Here's the drawing with two shaded views (mm, measured from the low corner). I have some questions. Round coordinates to 2 decimals unless told otherwise and drop trailing zeros. Write each loop counter-clockwise with the first axis right and the second up, starting at its lowest first coordinate (ties: lowest second). Pieces come first, ordered by that corner, then holes.
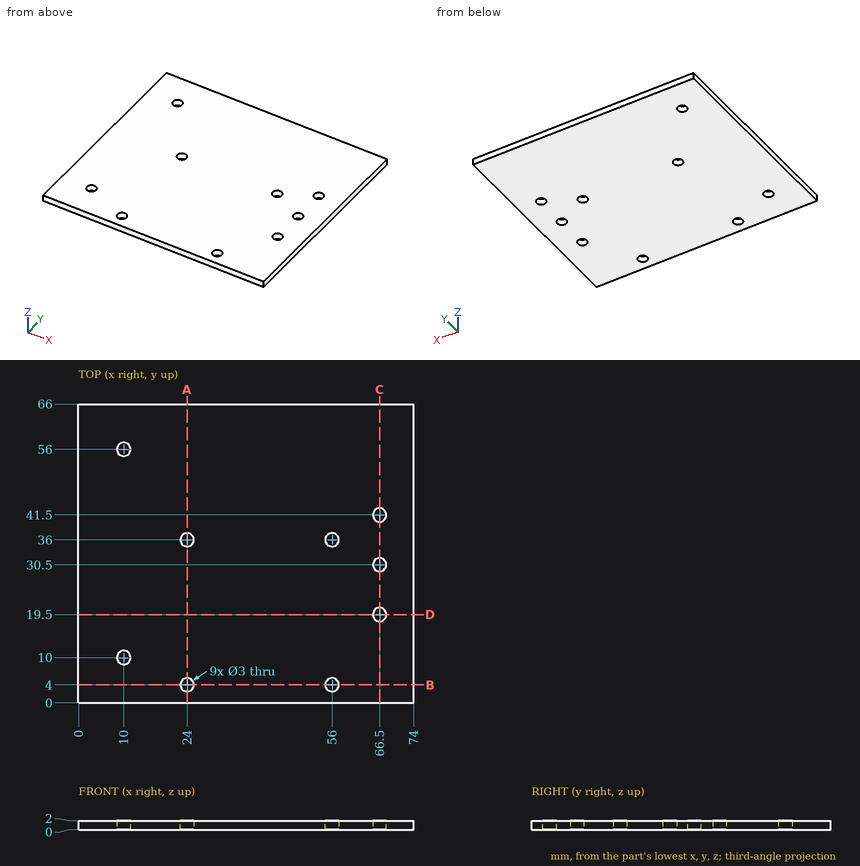
Q1. If I drill on L1, parallel to Y at x = 56, z = 0.6; L2, parallel to Y at x = 10, z = 1.4; L3, parallel to Y at x = 66.5, z = 1.25, over which ranges is the centre line in solid material (lowest first)?
Q2. Imagine slicing it at B-B, the plane y = 4. Write out the boundary of the cut face in (x, z).
Q3. Imagine slicing it at D-D, the plane y = 19.5. Write out the boundary of the cut face in (x, z).
Q4. Imagine slicing it at A-A, the plane x = 24. Write out the boundary of the cut face in (y, z), then the cut area to 3 significant figures.
Q5. I'm going to push a flat-ended pin straight in: pin 1 Ø3 at (x, y) = (46, 22.5) entering from -Z. Where does the tip first touch, or does it pass through?
Q6. Imagine slicing it at C-C, the plane x = 66.5. Write out the boundary of the cut face in (y, z), then the cut area to 3 significant figures.
Results found:
1. L1: y = 0 to 2.5, 5.5 to 34.5, 37.5 to 66
1. L2: y = 0 to 8.5, 11.5 to 54.5, 57.5 to 66
1. L3: y = 0 to 18, 21 to 29, 32 to 40, 43 to 66
2. outline: (0, 0) - (22.5, 0) - (22.5, 2) - (0, 2) - close; (25.5, 0) - (54.5, 0) - (54.5, 2) - (25.5, 2) - close; (57.5, 0) - (74, 0) - (74, 2) - (57.5, 2) - close
3. outline: (0, 0) - (65, 0) - (65, 2) - (0, 2) - close; (68, 0) - (74, 0) - (74, 2) - (68, 2) - close
4. outline: (0, 0) - (2.5, 0) - (2.5, 2) - (0, 2) - close; (5.5, 0) - (34.5, 0) - (34.5, 2) - (5.5, 2) - close; (37.5, 0) - (66, 0) - (66, 2) - (37.5, 2) - close
4. area: 120 mm2
5. pin 1: stops at z = 0
6. outline: (0, 0) - (18, 0) - (18, 2) - (0, 2) - close; (21, 0) - (29, 0) - (29, 2) - (21, 2) - close; (32, 0) - (40, 0) - (40, 2) - (32, 2) - close; (43, 0) - (66, 0) - (66, 2) - (43, 2) - close
6. area: 114 mm2
